Geometry: final body of the model. Coordinates: model frame, mm. A direction names the side the tool comes from. Coordinates: 2 decimals unless noted, no trailing zeros. Write each loop counter-clockwise with the first axis right and the second up, starting at its lowest first coordinate (ties: lowest second). Pieces come first, ordered by that corner, then holes. Notation, with made-up numbers: M -38.5,47 L 13.5,47 A29 cw 13.5,78 Z; hole C 8.5,-29.75 d4. An arc over 180 degrees is marked long. Write item = value, one per line. Start each with the question number.
Item 1: Ray query, L1, parallel to Z at x = 0, y = 10.75; L2, parallel to X at y = 7, z = 67; L3, parallel to X at y = 0.5, z = 10. Return the intervals inside material, ascending. Write a range as [from, to].
Item 2: Section B-B on z = 75. Output: boundary loops of the cut face in (x, y), plus the area to 3 significant figures.
Item 3: Reachability of faces 1 (the flat face through (0, 0, 80)), 2 (the flat face through (0, 4.5, 67)) from +Z, -Z, +X, -X, +Y, -Y: full face, straight path, thin tool, end or side. Return the list, or none.
Item 4: Pull-direction query (X, two-part tool) for faces 3 (the flat face through (0, 0, 0)), 4 (the cylindrical face through (5.77, -11.09, 39.45)), 5 (the cylindrical face through (0, 9, 63)); classes: +X half, -X half, draft (parallel to the pull), parting line (faces both ways), or undercut.
Item 5: First-contact query: pin 1 Ø4 at (x, z) = (5, 47.5) entering from +Y; pin 2 Ø1.5 at (y, z) = (-8, 10.5) entering from +X; pin 3 Ø8 at (y, z) = (-8.5, 61.5) entering from +X. Flat tips, straight axial feed; report the tip coordinate or a pass-through.
Item 6: Section A-A on x = 0. Output: boundary loops of the cut face in (y, z), plus the area to 3 significant figures.
Item 7: Section C-C on z = 65. Output: boundary loops of the cut face in (x, y).
from build123d import *

# Parameters (mm, degrees)
SKETCH1_R           = 12.5
BOSS_EXTRUDE4_DEPTH = 80
SKETCH5_R           = 4
CUT_EXTRUDE4_DEPTH  = 8
CHAMFER5_SIZE       = 1


with BuildPart() as part:
    # Sketch1 → Boss-Extrude4 (new body)
    with BuildSketch(Plane.XY):
        Circle(SKETCH1_R)
    extrude(amount=BOSS_EXTRUDE4_DEPTH)

    # Sketch5 → Cut-Extrude4 (cut)
    with BuildSketch(Plane(origin=(0, 12.5, 0), x_dir=(1, 0, 0), z_dir=(0, 1, 0))):
        with Locations(Location((0, -67, 0), (0, 0, 270))):
            Circle(SKETCH5_R)
    extrude(amount=-CUT_EXTRUDE4_DEPTH, mode=Mode.SUBTRACT)

    # Chamfer5
    chamfer5_edges = [part.edges().sort_by_distance(p)[0] for p in [
        (-12.5, 0, 0),
        (-12.5, 0, 80),
    ]]
    chamfer(chamfer5_edges, length=CHAMFER5_SIZE)


solid = part.part
Responses:
q1.L1 = [0, 63], [71, 80]
q1.L2 = [-10.36, -4], [4, 10.36]
q1.L3 = [-12.49, 12.49]
q2.outline = C 0,0 d25
q2.area = 491 mm²
q3.face_1 = +Z, +X, -X, +Y, -Y
q3.face_2 = +Y
q4.face_3 = draft
q4.face_4 = parting line
q4.face_5 = undercut
q5.pin_1 = 12.13
q5.pin_2 = 10.18
q5.pin_3 = 11.66
q6.outline = M -12.5,1 L -11.5,0 L 11.5,0 L 12.5,1 L 12.5,63 L 4.5,63 L 4.5,71 L 12.5,71 L 12.5,79 L 11.5,80 L -11.5,80 L -12.5,79 Z
q6.area = 1,930 mm²
q7.outline = M -3.46,4.5 L -3.46,12.01 A12.5 ccw long 3.46,12.01 L 3.46,4.5 Z
